Could you check a few things on this model? Use its own coordinates, in mm. A direction names the side the tool comes from. Round coordinates to 2 decimals unless told otherwise and drop trailing zeros. Order: outer loops, then holes, each group sorted by start corner. A loop starts at its lowest first (then second) coordinate and runs counter-clockwise, first axis right, second up.
```python
from build123d import *

# Parameters (mm, degrees)
SKETCH1_W            = 20
SKETCH1_H            = 46.382365304
SKETCH1_R            = 2.6
SKETCH1_R_2          = 1.75
SKETCH1_R_3          = 2.75
BOSS_EXTRUDE2_DEPTH  = 2
SKETCH2_R            = 2.6
BOSS_EXTRUDE3_DEPTH  = 10
SKETCH4_R            = 1.75
BOSS_EXTRUDE5_DEPTH  = 2
SKETCH5_R            = 4.5
CUT_EXTRUDE1_DEPTH   = 5
SKETCH3_W            = 18
SKETCH3_H            = 8.25
SKETCH3_R            = 1.75
BOSS_EXTRUDE9_DEPTH  = 7.6
SKETCH8_R            = 2.55
CUT_EXTRUDE3_DEPTH   = 3.8
CHAMFER5_SIZE2       = 3.8
CHAMFER5_SIZE        = 0.105
CHAMFER6_SIZE        = 6
CHAMFER7_SIZE        = 2
SKETCH9_W            = 2
SKETCH9_H            = 6.5
BOSS_EXTRUDE10_DEPTH = 1.5
SKETCH10_W           = 2
SKETCH10_H           = 0.75
BOSS_EXTRUDE11_DEPTH = 6.1
CHAMFER8_SIZE        = 1
SKETCH13_R           = 1.875965007
BOSS_EXTRUDE14_DEPTH = 7.6
SKETCH12_R           = 1.5
BOSS_EXTRUDE15_DEPTH = 1.6
SKETCH14_W           = 6
SKETCH14_H           = 4
BOSS_EXTRUDE16_DEPTH = 2
CHAMFER9_SIZE        = 2


# Some blends are built 0.0001 mm under size
with BuildPart() as part:
    # Sketch1 → Boss-Extrude2 (new body)
    with BuildSketch(Plane.XY):
        with Locations((-1.1970966, -0.016031908)):
            Rectangle(SKETCH1_W, SKETCH1_H)
        with Locations((-1.1970966, 16.983968092)):
            Circle(SKETCH1_R, mode=Mode.SUBTRACT)
        with Locations((-1.1970966, 7)):
            Circle(SKETCH1_R_2, mode=Mode.SUBTRACT)
        with Locations((-1.1970966, 0)):
            Circle(SKETCH1_R_3, mode=Mode.SUBTRACT)
    extrude(amount=BOSS_EXTRUDE2_DEPTH)

    # Sketch2 → Boss-Extrude3 (add)
    with BuildSketch(Plane.XY.offset(2)):
        Polygon((-11.1970966, 23.175150744), (-11.1970966, -23.20721456), (8.8029034, -23.20721456), (8.8029034, -11.5), (-9.1970966, -11.5), (-9.1970966, 11.5), (8.8029034, 11.5), (8.8029034, 23.175150744), align=None)
        with Locations((-1.1970966, 16.983968092)):
            Circle(SKETCH2_R, mode=Mode.SUBTRACT)
    extrude(amount=BOSS_EXTRUDE3_DEPTH)

    # Sketch4 → Boss-Extrude5 (add)
    with BuildSketch(Plane(origin=(0, 0, 0), x_dir=(-1, 0, 0), z_dir=(0, 0, -1))):
        with Locations((1.1970966, 7)):
            Circle(SKETCH4_R)
    extrude(amount=-BOSS_EXTRUDE5_DEPTH)

    # Sketch5 → Cut-Extrude1 (cut)
    with BuildSketch(Plane(origin=(0, 0, 0), x_dir=(-1, 0, 0), z_dir=(0, 0, -1))):
        with Locations((1.1970966, 16.983968092)):
            Circle(SKETCH5_R)
    extrude(amount=-CUT_EXTRUDE1_DEPTH, mode=Mode.SUBTRACT)

    # Sketch3 → Boss-Extrude9 (add)
    # profile 1 of 2: a face of its own
    with BuildSketch(Plane.XY.offset(2)):
        with Locations((-0.1970966, -7.375)):
            Rectangle(SKETCH3_W, SKETCH3_H)
        with Locations(Location((-1.1970966, -7, 0), (0, 0, 180))):
            Circle(SKETCH3_R, mode=Mode.SUBTRACT)
    # profile 2 of 2: a face of its own
    with BuildSketch(Plane.XY.offset(2)):
        with Locations((-0.1970966, 7.375)):
            Rectangle(SKETCH3_W, SKETCH3_H)
        with Locations(Location((-1.1970966, 7, 0), (0, 0, 180))):
            Circle(SKETCH3_R, mode=Mode.SUBTRACT)
    extrude(amount=BOSS_EXTRUDE9_DEPTH)

    # Sketch8 → Cut-Extrude3 (cut)
    with BuildSketch(Plane.XY.offset(9.6)):
        with Locations((-1.1970966, 7)):
            Circle(SKETCH8_R)
    extrude(amount=-CUT_EXTRUDE3_DEPTH, mode=Mode.SUBTRACT)

    # Chamfer5
    chamfer5_edges = [part.edges().sort_by_distance(p)[0] for p in [
        (-3.7470966, 7, 9.6),
    ]]
    chamfer5_side = [part.faces().sort_by_distance(p)[0] for p in [
        (-3.7491966, 7, 9.6),
    ]]
    chamfer(chamfer5_edges, length=CHAMFER5_SIZE - 0.0001, length2=CHAMFER5_SIZE2 - 0.0001, reference=chamfer5_side[0])  # a hair under: the kernel refuses the full size

    # Chamfer6
    # the kernel refuses this chamfer: 6 mm, written as the material it takes off along each edge
    with BuildSketch(Plane(origin=(-26.627194528, 23.175150744, 0), x_dir=(0, 0.027495876610586202, 0.9996219169112968), z_dir=(1, 0, 0)), Plane(origin=(24.233001328, -23.20721456, 0), x_dir=(0, -0.027495876610586202, 0.9996219169112968), z_dir=(-1, 0, 0))) as chamfer6_piece_1:
        Polygon((CHAMFER6_SIZE * 0.999621916911, CHAMFER6_SIZE * 0.0274958766106), (-CHAMFER6_SIZE * 0.0274958766106, CHAMFER6_SIZE * 0.999621916911), (0, 0), align=None)
    extrude(amount=50.860195856, mode=Mode.SUBTRACT)

    # Chamfer7
    chamfer7_edges = [part.edges().sort_by_distance(p)[0] for p in [
        (-11.1970966, -0.016031908, 0),
        (8.8029034, -0.016031908, 0),
        (8.8029034, -20.20721456, 3),
        (8.8029034, 20.175150744, 3),
        (-11.1970966, -20.20721456, 3),
        (-11.1970966, 20.175150744, 3),
        (-11.1970966, -23.20721456, 9),
        (-11.1970966, 23.175150744, 9),
        (8.8029034, 23.175150744, 9),
        (8.8029034, -23.20721456, 9),
    ]]
    chamfer(chamfer7_edges, length=CHAMFER7_SIZE - 0.0001)  # a hair under: the kernel refuses the full size

    # Sketch9 → Boss-Extrude10 (add)
    with BuildSketch(Plane.XY.offset(2)):
        with Locations((7.8029034, 0)):
            Rectangle(SKETCH9_W, SKETCH9_H)
    extrude(amount=BOSS_EXTRUDE10_DEPTH)

    # Sketch10 → Boss-Extrude11 (add)
    with BuildSketch(Plane.XY.offset(3.5)):
        with Locations((7.8029034, 2.875)):
            Rectangle(SKETCH10_W, SKETCH10_H)
        with Locations((7.8029034, -2.875)):
            Rectangle(SKETCH10_W, SKETCH10_H)
    extrude(amount=BOSS_EXTRUDE11_DEPTH)

    # Chamfer8
    chamfer8_edges = [part.edges().sort_by_distance(p)[0] for p in [
        (6.8029034, -3.25, 5.8),
        (6.8029034, 0, 2),
        (6.8029034, 3.25, 5.8),
    ]]
    chamfer(chamfer8_edges, length=CHAMFER8_SIZE)

    # Sketch13 → Boss-Extrude14 (add)
    with BuildSketch(Plane.XY.offset(2)):
        with Locations((-1.1970966, -7)):
            Circle(SKETCH13_R)
    extrude(amount=BOSS_EXTRUDE14_DEPTH)

    # Sketch12 → Boss-Extrude15 (add)
    with BuildSketch(Plane.XY.offset(9.6)):
        with Locations((-1.1970966, -7)):
            Circle(SKETCH12_R)
    extrude(amount=BOSS_EXTRUDE15_DEPTH)

    # Sketch14 → Boss-Extrude16 (add)
    with BuildSketch(Plane.XY.offset(12)):
        with Locations((-1.1970966, -21.20721456)):
            Rectangle(SKETCH14_W, SKETCH14_H)
    extrude(amount=BOSS_EXTRUDE16_DEPTH)

    # Chamfer9
    chamfer9_edges = [part.edges().sort_by_distance(p)[0] for p in [
        (-1.1970966, -19.20721456, 14),
    ]]
    chamfer(chamfer9_edges, length=CHAMFER9_SIZE - 0.0001)  # a hair under: the kernel refuses the full size


solid = part.part
```
Q1. Imagine slicing it at A-A, the plane y = 0. Please give me the cut outline in (x, z).
Q2. I need wall thicknesses on L1, parallel to Y at x = 4.5, z = 11; L2, parallel to Z at x = 8.25, y = -4.5; L3, parallel to X at y = 5.5, z = 6.5. Which ranges of each line are inside material? Lowest first, please.
Q3. For P1, Ø5.5, axis at x = -0.5, y = 7, coming from the +Z side; P2, Ø2.5, axis at x = -2.5, y = 16, coming from the -Z side; P3, Ø8, axis at x = 2.5, y = -4.5, coming from the +Z side, each with a flat end and sliding along its axis, tell me the tip position at first contact or that it passes through.
Q4. We'd pull the mould along Y, two halves only. Please class faces 1 (the flat face through (-10, 0, 12)), 2 (the flat face through (0, -9, 9.6)), 3 (the flat face through (-9.197, 0, 8)), 4 (the flat face through (-10.21, 22.16, 9.04)): released by +Y, released by -Y, zero draft, split by the parting line, or undercut.
Q5. Imagine slicing it at B-B, the plane x = -6.5. Please give me the cut outline in (y, z), then the cut area to 3 significant figures.
Q6. Imagine slicing it at D-D, the plane z = 1.25. Please give me the cut outline in (x, y).
Q7. For faces 5 (the flat face through (7.79, 19.52, 3.74)), 6 (the cylindrical face through (-2.005, 8.553, 3.873)), which set-ups out of +Z, -Z, +X, -X, +Y, -Y let a thin tool reach every point of the face, with its end or its side?
Q8. Imagine slicing it at C-C, the plane y = -10. Please give me the cut outline in (x, z).
Filled in:
1. outline: (-11.2, 2) - (-9.2, 0) - (-3.95, 0) - (-3.95, 2) - (-9.2, 2) - (-9.2, 12) - (-11.2, 12) - close; (1.55, 0) - (6.8, 0) - (8.8, 2) - (8.8, 3.5) - (6.8, 3.5) - (6.8, 3) - (5.8, 2) - (1.55, 2) - close
2. L1: y = -23.21 to -11.5, 11.5 to 23.18
2. L2: z = 1.45 to 9.6
2. L3: x = -11.2 to -3.28, 0.89 to 8.8
3. P1: stops at z = 9.6
3. P2: stops at z = 5
3. P3: stops at z = 11.2
4. face 1: zero draft
4. face 2: undercut
4. face 3: undercut
4. face 4: released by +Y
5. outline: (-23.21, 6) - (-17.21, 0) - (17.18, 0) - (23.18, 6) - (23.18, 12) - (11.5, 12) - (11.5, 9.6) - (3.25, 9.6) - (3.25, 2) - (-3.25, 2) - (-3.25, 9.6) - (-11.5, 9.6) - (-11.5, 12) - (-23.21, 12) - close
5. area: 416 mm2
6. outline: (-10.45, -16.69) - (-9.2, -18.46) - (6.8, -18.46) - (8.05, -16.69) - (8.05, 16.66) - (6.8, 18.43) - (3.07, 18.43) arc R4.5 cw (long way) to (-5.46, 18.43) - (-9.2, 18.43) - (-10.45, 16.66) - close; hole circle Ø5.5 at (-1.2, 0)
7. face 5: -Z, +X, +Y
7. face 6: +Z
8. outline: (-11.2, 2) - (-9.2, 0) - (6.8, 0) - (8.8, 2) - (8.8, 9.6) - (-9.2, 9.6) - (-9.2, 12) - (-11.2, 12) - close
